Work out the finished part from the listing and answer in its coordinate system (mm). A direction names the side the tool comes from. Round coordinates to 2 decimals unless told otherwise and drop trailing zeros. Order: outer loops, then holes, each group sorted by start corner. A loop starts at its lowest first (then second) coordinate and runs counter-clockwise, first axis right, second up. Notation, with made-up numbers: (14, 89.5) - (40, 89.5) arc R33 cw to (40, 125.5) - close; hole circle Ø10 at (24.25, 49.25). An arc over 180 degrees is marked (long way). Put each result on its own line as item: value.
Autodesk Inventor part; units mm, degrees
ref_plane "YZ Plane" through (0, 0, 0) normal (1, 0, 0) x (0, 1, 0)
ref_plane "XZ Plane" through (0, 0, 0) normal (0, 1, 0) x (-1, 0, 0)
ref_plane "XY Plane" through (0, 0, 0) normal (0, 0, 1) x (1, 0, 0)
sketch "Sketch1" plane through (0, 0, 0) normal (0, 1, 0) x (-1, 0, 0)
  line L0 (0, 0) -> (28.575, 0)
  line L1 (28.575, 0) -> (0, 0)
  line L2 (0, 0) -> (-14.2875, -24.7467)
  line L3 (0, 0) -> (28.575, 0) construction
  line L4 (0, 0) -> (-14.2875, 24.7467)
  line L5 (0, 0) -> (28.575, 0) construction
  circle A0 centre (28.575, 0) radius 2.54
  circle A1 centre (-14.2875, -24.7467) radius 2.54
  circle A2 centre (-14.2875, 24.7467) radius 2.54
  circle A3 centre (0, 0) radius 3.175
  circle A4 centre (0, 0) radius 6.35
  line L6 (-1.5875, -2.7496) -> (0, 0)
  line L7 (0, 0) -> (-6.35, 0)
  circle A5 centre (-14.2875, 24.7467) radius 3.81
  circle A6 centre (28.575, 0) radius 3.81
  circle A7 centre (-14.2875, -24.7467) radius 3.81
  line L8 (30.6811, 3.175) -> (-12.1814, 27.9217)
  line L9 (28.2054, -3.792) -> (-10.8187, -26.3226)
  line L10 (-18.0975, 24.7467) -> (-18.0975, -24.7467)
  line L11 (0, 0) -> (5.0525, -8.8146)
  line L12 (0, 0) -> (5.1463, 8.7602)
  line L13 (0, 0) -> (-10.16, 0)
  arc A8 (28.2054, -3.792) -> (-10.8187, -26.3226) centre (24.4473, -42.344) ccw
  arc A9 (-10.8187, 26.3226) -> (28.2054, 3.792) centre (24.4473, 42.344) ccw
  arc A10 (-17.3867, -22.5305) -> (-17.3867, 22.5305) centre (-48.8947, 0) ccw
  point P0 (5.1074, 8.7829)
  point P1 (-10.16, 0.0317)
  point P2 (30.2716, 3.4114)
  point P3 (28.2054, 3.792)
  point P4 (-10.8187, 26.3226)
  point P5 (-17.3867, 22.5305)
  point P6 (-17.3867, -22.5305)
  dimension "d9" = 6.35
  dimension "d41" = 12.7
  dimension "d0" = 28.575
  dimension "d1" = 28.575
  dimension "d2" = 120
  dimension "d3" = 28.575
  dimension "d4" = 120
  dimension "d5" = 5.08
  dimension "d6" = 5.08
  dimension "d7" = 5.08
  dimension "d42" = 7.62
  dimension "d43" = 7.62
  dimension "d44" = 7.62
  dimension "d47" = 10.16
  dimension "d48" = 10.16
  dimension "d49" = 10.16
  dimension "d52" = 360
extrude "Extrusion4" add sketch "Sketch1" along normal blind 12.7 contours A3 L12 A4 L0 | L0 A4 L11 A3 | A3 L11 A4 L2 | L2 A4 L7 A3 | A3 L7 A4 L4 | L4 A4 L12 A3 | A4 L12 A9 A6 L0 | L0 A6 A8 L11 A4 | A4 L11 A8 A7 L2 | L2 A7 A10 L13 A4 | A4 L13 A10 A5 L4 | L4 A5 A9 L12 A4 | A6 L8 | A7 | A5 picked at (31.8987, 0.5122)
sketch "Sketch21" plane through (0, 12.7, 0) normal (0, 1, 0) x (1, 0, 0)
  circle A0 centre (-28.575, 0) radius 2.54
  arc A1 (-28.2054, 3.792) -> (10.8187, 26.3226) centre (-24.4473, 42.344) ccw
  arc A2 (10.8187, -26.3226) -> (-28.2054, -3.792) centre (-24.4473, -42.344) ccw
  arc A3 (-28.2054, 3.792) -> (10.8187, 26.3226) centre (-24.4473, 42.344) ccw
  arc A4 (-28.2054, 3.792) -> (-30.6811, -3.175) centre (-28.575, 0) ccw
  line L0 (-30.6811, -3.175) -> (-30.2716, -3.4114)
  arc A5 (-30.2716, -3.4114) -> (-28.2054, -3.792) centre (-28.575, 0) ccw
  arc A6 (10.8187, -26.3226) -> (-28.2054, -3.792) centre (-24.4473, -42.344) ccw
  arc A7 (10.8187, -26.3226) -> (17.3867, -22.5305) centre (14.2875, -24.7467) ccw
  arc A8 (17.3867, 22.5305) -> (17.3867, -22.5305) centre (48.8947, 0) ccw
  arc A9 (17.3867, 22.5305) -> (10.8187, 26.3226) centre (14.2875, 24.7467) ccw
  circle A10 centre (-28.575, 0) radius 2.54
  circle A11 centre (0, 0) radius 3.175
  circle A12 centre (14.2875, -24.7467) radius 2.54
  circle A13 centre (14.2875, 24.7467) radius 2.54
  line L1 (0, 0) -> (-13.6784, 0)
  line L2 (-13.6784, 0) -> (-28.575, 0)
  line L3 (0, 0) -> (-10.795, 0)
  line L4 (-10.795, 0) -> (-10.795, 6.095)
  arc A14 (-28.2054, 3.792) -> (10.8187, 26.3226) centre (-24.4473, 42.344) ccw
  line L5 (-10.795, 0) -> (-10.795, -6.095)
  point P0 (10.8187, -26.3226)
  point P1 (10.8187, 26.3226)
  dimension "d107" = 10.795
sketch "Sketch22" plane through (0, 0, 0) normal (0, -1, 0) x (1, 0, 0)
  line L0 (0, 0) -> (-17.145, 0)
  line L1 (-17.145, 0) -> (-17.145, -4.3038)
  arc A0 (10.8187, -26.3226) -> (-28.2054, -3.792) centre (-24.4473, -42.344) ccw
  line L2 (-17.145, 0) -> (-17.145, 4.3038)
  arc A1 (-28.2054, 3.792) -> (10.8187, 26.3226) centre (-24.4473, 42.344) ccw
  arc A2 (10.8187, -26.3226) -> (-28.2054, -3.792) centre (-24.4473, -42.344) ccw
  arc A3 (10.8187, -26.3226) -> (17.3867, -22.5305) centre (14.2875, -24.7467) ccw
  arc A4 (17.3867, 22.5305) -> (17.3867, -22.5305) centre (48.8947, 0) ccw
  arc A5 (17.3867, 22.5305) -> (10.8187, 26.3226) centre (14.2875, 24.7467) ccw
  arc A6 (-28.2054, 3.792) -> (10.8187, 26.3226) centre (-24.4473, 42.344) ccw
  arc A7 (-28.2054, 3.792) -> (-30.2716, 3.4114) centre (-28.575, 0) ccw
  line L3 (-30.6811, 3.175) -> (-30.2716, 3.4114)
  arc A8 (-30.6811, 3.175) -> (-28.2054, -3.792) centre (-28.575, 0) ccw
  circle A9 centre (-28.575, 0) radius 2.54
  circle A10 centre (0, 0) radius 3.175
  circle A11 centre (14.2875, 24.7467) radius 2.54
  circle A12 centre (14.2875, -24.7467) radius 2.54
  point P0 (10.8187, -26.3226)
  point P1 (10.8187, 26.3226)
  dimension "d108" = 17.145
extrude "Extrusion10" cut sketch "Sketch22" against normal blind 6.35 contours L2 A1 A5 A4 A3 A0 L1
extrude "Extrusion11" cut sketch "Sketch21" against normal blind 6.35 contours A1 A9 A8 A7 A2 L5 L4
sketch "Sketch23" plane through (0, 12.7, 0) normal (0, 1, 0) x (1, 0, 0)
  point P0 (0, 0)
sketch "Sketch24" plane through (0, 6.35, 0) normal (0, -1, 0) x (1, 0, 0)
  line L0 (-17.145, -4.3038) -> (-17.145, 4.3038)
  line L1 (-17.145, 0) -> (-10.795, 0)
  line L2 (-10.795, -6.095) -> (-10.795, 6.095)
  line L3 (-13.97, 0) -> (-13.97, 5.0532)
  arc A0 (-17.145, 4.3038) -> (-10.795, 6.095) centre (-24.4473, 42.344) ccw
  line L4 (-13.97, 0) -> (-13.97, -5.0532)
  arc A1 (-10.795, -6.095) -> (-17.145, -4.3038) centre (-24.4473, -42.344) ccw
  point P0 (0, 0)
hole "Hole8" at (-13.97, 6.35, 0) direction (0, 1, 0) diameter 2.1129 depth 7.7978
properties part number "stability copy2"
1) A cutting plane is placed at D-D on y = 3. Write down the section's boundary in (x, z) (3 decimals).
Findings below:
outline: (-30.681, 3.175) arc R3.81 ccw to (-28.205, -3.792) arc R38.735 cw to (-17.145, -4.304) - (-17.145, 4.304) arc R38.735 cw to (-28.205, 3.792) arc R3.81 ccw to (-30.272, 3.411) - close; hole circle Ø5.08 at (-28.575, 0)
2) A cutting plane is placed at B-B on x = -13.97. Write down the section's boundary in (y, z).
Findings below:
outline: (6.35, -5.05) - (12.7, -5.05) - (12.7, -1.06) - (6.35, -1.06) - close; (6.35, 1.06) - (12.7, 1.06) - (12.7, 5.05) - (6.35, 5.05) - close
3) A cutting plane is placed at A-A on z = 0. Write down the section's boundary in (x, y) (3 decimals), then the cut area to 3 significant figures.
Findings below:
outline: (-32.385, 0) - (-31.115, 0) - (-31.115, 12.7) - (-32.385, 12.7) - close; (-26.035, 0) - (-17.145, 0) - (-17.145, 6.35) - (-15.026, 6.35) - (-15.026, 12.7) - (-26.035, 12.7) - close; (-12.914, 6.35) - (-10.795, 6.35) - (-10.795, 12.7) - (-12.914, 12.7) - close
area: 156 mm2
4) A cutting plane is placed at C-C on y = 10. Write down the section's boundary in (x, z) (3 decimals), then the cut area to 3 significant figures.
Findings below:
outline: (-30.681, 3.175) arc R3.81 ccw to (-28.205, -3.792) arc R38.735 cw to (-10.795, -6.095) - (-10.795, 6.095) arc R38.735 cw to (-28.205, 3.792) arc R3.81 ccw to (-30.272, 3.411) - close; hole circle Ø5.08 at (-28.575, 0); hole circle Ø2.113 at (-13.97, 0)
area: 150 mm2
5) Given pin 1 Ø5 at (x, y) = (-27, 9) entering from -Z; pin 2 Ø4 at (x, z) = (-28.575, 0) entering from -Y; pin 3 Ø3 at (y, z) = (2.5, -0.5) entering from +X (3 decimals), each flat-ended and moving along its own axis, determine where each tip first touches the part or whether it passes through.
Findings below:
pin 1: stops at z = -3.81
pin 2: passes through
pin 3: stops at x = -17.145
6) For faces 4 (the flat face through (-12.6, 6.35, 0.1)), 5 (the cylindrical face through (-21.202, 6.261, -3.745)), determine the directions among +Z, -Z, +X, -X, +Y, -Y from which every point of the face is accessible in a straight line to the end or side of a thin tool.
Findings below:
face 4: +Z, -Z, +X, -Y
face 5: -Z, +Y, -Y
7) For a pull along Z with two mould halves and no side action, classify faces 1 (the cylindrical face through (-26.037, 6.261, -0.112)), 2 (the cylindrical face through (-21.449, 6.261, 3.726)), 3 (the cylindrical face through (-32.188, 6.261, -1.209)) as pulls with the +Z half, pulls with the -Z half, needs draft (parallel to the pull), parting line crosses it, or undercut.
Findings below:
face 1: undercut
face 2: pulls with the +Z half
face 3: parting line crosses it
8) Straight lines are drawn through the part: L1, parallel to X at y = 10, z = 0 (3 decimals); L2, parallel to Z at x = -28.75, y = 10.25; L3, parallel to X at y = 4, z = 0 (3 decimals). For each, find the intervals that lie inside material, in ascending order. Write a range as from..to.
Findings below:
L1: x = -32.385..-31.115, -26.035..-15.026, -12.914..-10.795
L2: z = -3.81..-2.53, 2.53..3.81
L3: x = -32.385..-31.115, -26.035..-17.145
